Input: part model. Units: mm. Frame: model coordinates. Round coordinates to 2 decimals unless told otherwise and drop trailing zeros.
1) Draft query along X for faces 1 (the face through (-16.9, 9.4, 493)), 2 (the face through (-19, -2, 0)), 3 (the face through (-3.646, -3.826, 493)), 4 (the face through (-7.086, 5.552, 493)). Return one class per face: pulls with the +X half, pulls with the -X half, needs draft (parallel to the pull), parting line crosses it, or undercut.
2) First-contact query: pin 1 (5 mm diameter, centred on x = -14, z = 307, fed in from -Y); pin 2 (1 mm diameter, centred on x = -3.5, z = 527.5, fed in from +Y); pin 3 (1 mm diameter, centred on x = -28.5, z = 569, fed in from -Y); pin 4 (2 mm diameter, centred on x = -14.5, y = 5, fed in from -Z). Flat tips, straight axial feed; report the tip coordinate or a pass-through.
3) Ray query, line 1 along X through (y, z) = (-14, 844); line 2 along Y through (x, z) = (-14.5, 451.5); line 3 along X through (y, z) = (-12, 358). Return the intervals inside material, ascending.
4) Section A-A, the plane z = 912.5. State how many separate pieces and enclosed holes the cut face has, and give its area (3 significant figures).
from build123d import *

# Parameters (mm, degrees)
SKETCH_1_R      = 3.4
EXTRUDE_1_DEPTH = 1000


with BuildPart() as part:
    # 草图1 → 凸台-拉伸1 (new body)
    with BuildSketch(Plane.XY):
        with BuildLine():
            Line((-29.957449905, -7.030330124), (-29.957449905, -14.430330124))
            ThreePointArc((-29.957449905, -14.430330124), (-29.225216858, -16.198097077), (-27.457449905, -16.930330124))
            Line((-27.457449905, -16.930330124), (-20.057449905, -16.930330124))
            Line((-20.057449905, -16.930330124), (-20.057449905, -16.130330124))
            ThreePointArc((-20.057449905, -16.130330124), (-19.998871261, -15.988908768), (-19.857449905, -15.930330124))
            Line((-19.857449905, -15.930330124), (-19.057449905, -15.930330124))
            Line((-19.057449905, -15.930330124), (-19.057449905, -15.030330124))
            ThreePointArc((-19.057449905, -15.030330124), (-19.145317871, -14.818198089), (-19.357449905, -14.730330124))
            Line((-19.357449905, -14.730330124), (-22.907449905, -14.730330124))
            ThreePointArc((-22.907449905, -14.730330124), (-23.11958194, -14.642462158), (-23.207449905, -14.430330124))
            Line((-23.207449905, -14.430330124), (-23.207449905, -11.735965042))
            Line((-23.207449905, -11.735965042), (-19.201814987, -7.730330124))
            Line((-19.201814987, -7.730330124), (-10.713084824, -7.730330124))
            Line((-10.713084824, -7.730330124), (-6.707449905, -11.735965042))
            Line((-6.707449905, -11.735965042), (-6.707449905, -14.430330124))
            ThreePointArc((-6.707449905, -14.430330124), (-6.795317871, -14.642462158), (-7.007449905, -14.730330124))
            Line((-7.007449905, -14.730330124), (-10.557449905, -14.730330124))
            ThreePointArc((-10.557449905, -14.730330124), (-10.76958194, -14.818198089), (-10.857449905, -15.030330124))
            Line((-10.857449905, -15.030330124), (-10.857449905, -15.930330124))
            Line((-10.857449905, -15.930330124), (-10.057449905, -15.930330124))
            ThreePointArc((-10.057449905, -15.930330124), (-9.916028549, -15.988908768), (-9.857449905, -16.130330124))
            Line((-9.857449905, -16.130330124), (-9.857449905, -16.930330124))
            Line((-9.857449905, -16.930330124), (-2.457449905, -16.930330124))
            ThreePointArc((-2.457449905, -16.930330124), (-0.689682952, -16.198097077), (0.042550095, -14.430330124))
            Line((0.042550095, -14.430330124), (0.042550095, -11.930330124))
            ThreePointArc((0.042550095, -11.930330124), (-7.279780376, 5.747339406), (-24.957449905, 13.069669876))
            Line((-24.957449905, 13.069669876), (-27.457449905, 13.069669876))
            ThreePointArc((-27.457449905, 13.069669876), (-29.225216858, 12.337436829), (-29.957449905, 10.569669876))
            Line((-29.957449905, 10.569669876), (-29.957449905, 3.169669876))
            Line((-29.957449905, 3.169669876), (-29.157449905, 3.169669876))
            ThreePointArc((-29.157449905, 3.169669876), (-29.016028549, 3.111091232), (-28.957449905, 2.969669876))
            Line((-28.957449905, 2.969669876), (-28.957449905, 2.169669876))
            Line((-28.957449905, 2.169669876), (-28.057449905, 2.169669876))
            ThreePointArc((-28.057449905, 2.169669876), (-27.845317871, 2.257537842), (-27.757449905, 2.469669876))
            Line((-27.757449905, 2.469669876), (-27.757449905, 6.019669876))
            ThreePointArc((-27.757449905, 6.019669876), (-27.66958194, 6.231801911), (-27.457449905, 6.319669876))
            Line((-27.457449905, 6.319669876), (-24.763084824, 6.319669876))
            Line((-24.763084824, 6.319669876), (-20.757449905, 2.314034958))
            Line((-20.757449905, 2.314034958), (-20.757449905, -6.174695205))
            Line((-20.757449905, -6.174695205), (-24.763084824, -10.180330124))
            Line((-24.763084824, -10.180330124), (-27.457449905, -10.180330124))
            ThreePointArc((-27.457449905, -10.180330124), (-27.66958194, -10.092462158), (-27.757449905, -9.880330124))
            Line((-27.757449905, -9.880330124), (-27.757449905, -6.330330124))
            ThreePointArc((-27.757449905, -6.330330124), (-27.845317871, -6.118198089), (-28.057449905, -6.030330124))
            Line((-28.057449905, -6.030330124), (-28.957449905, -6.030330124))
            Line((-28.957449905, -6.030330124), (-28.957449905, -6.830330124))
            ThreePointArc((-28.957449905, -6.830330124), (-29.016028549, -6.97175148), (-29.157449905, -7.030330124))
            Line((-29.157449905, -7.030330124), (-29.957449905, -7.030330124))
        make_face()
        with Locations((-14.957449905, -1.930330124)):
            Circle(SKETCH_1_R, mode=Mode.SUBTRACT)
        with BuildLine():
            Line((-9.632006825, 4.950747875), (-10.713084824, 3.869669876))
            Line((-10.713084824, 3.869669876), (-19.201814987, 3.869669876))
            Line((-19.201814987, 3.869669876), (-23.651814987, 8.319669876))
            Line((-23.651814987, 8.319669876), (-27.457449905, 8.319669876))
            ThreePointArc((-27.457449905, 8.319669876), (-27.66958194, 8.407537842), (-27.757449905, 8.619669876))
            Line((-27.757449905, 8.619669876), (-27.757449905, 10.569669876))
            ThreePointArc((-27.757449905, 10.569669876), (-27.66958194, 10.781801911), (-27.457449905, 10.869669876))
            Line((-27.457449905, 10.869669876), (-24.957449905, 10.869669876))
            ThreePointArc((-24.957449905, 10.869669876), (-16.743089868, 9.338527137), (-9.632006825, 4.950747875))
        make_face(mode=Mode.SUBTRACT)
        with BuildLine():
            Line((-27.932449905, -15.205330124), (-25.232449905, -15.205330124))
            ThreePointArc((-25.232449905, -15.205330124), (-25.020317871, -15.117462158), (-24.932449905, -14.905330124))
            Line((-24.932449905, -14.905330124), (-24.932449905, -12.205330124))
            ThreePointArc((-24.932449905, -12.205330124), (-25.020317871, -11.993198089), (-25.232449905, -11.905330124))
            Line((-25.232449905, -11.905330124), (-27.932449905, -11.905330124))
            ThreePointArc((-27.932449905, -11.905330124), (-28.14458194, -11.993198089), (-28.232449905, -12.205330124))
            Line((-28.232449905, -12.205330124), (-28.232449905, -14.905330124))
            ThreePointArc((-28.232449905, -14.905330124), (-28.14458194, -15.117462158), (-27.932449905, -15.205330124))
        make_face(mode=Mode.SUBTRACT)
        with BuildLine():
            Line((-8.076371906, 3.395112956), (-9.157449905, 2.314034958))
            Line((-9.157449905, 2.314034958), (-9.157449905, -6.174695205))
            Line((-9.157449905, -6.174695205), (-4.707449905, -10.624695205))
            Line((-4.707449905, -10.624695205), (-4.707449905, -14.430330124))
            ThreePointArc((-4.707449905, -14.430330124), (-4.61958194, -14.642462158), (-4.407449905, -14.730330124))
            Line((-4.407449905, -14.730330124), (-2.457449905, -14.730330124))
            ThreePointArc((-2.457449905, -14.730330124), (-2.245317871, -14.642462158), (-2.157449905, -14.430330124))
            Line((-2.157449905, -14.430330124), (-2.157449905, -11.930330124))
            ThreePointArc((-2.157449905, -11.930330124), (-3.688592644, -3.715970087), (-8.076371906, 3.395112956))
        make_face(mode=Mode.SUBTRACT)
    extrude(amount=EXTRUDE_1_DEPTH)


solid = part.part
Final values:
1. face 1: undercut
1. face 2: needs draft
1. face 3: undercut
1. face 4: pulls with the +X half
2. pin 1: stops at y = -7.73
2. pin 2: stops at y = 1.7
2. pin 3: stops at y = -16.87
2. pin 4: passes through
3. line 1: x = -29.96 to -28.23, -24.93 to -23.21, -6.71 to -4.71, -2.16 to 0.04
3. line 2: y = -7.73 to -5.3, 1.44 to 3.87, 8.33 to 10.78
3. line 3: x = -29.96 to -28.15, -25.01 to -23.21, -6.71 to -4.71, -2.16 to 0.04
4. separate pieces: 1
4. enclosed holes: 4
4. area: 337 mm2
